```python
from build123d import *

# Parameters (mm, degrees)
F0_R     = 12.7
F1_DEPTH = 20.32
F2_T     = -2.54
F3_R     = 0.889


with BuildPart() as f1:
    # F0 (on Front) → F1 (new body)
    with BuildSketch(Plane.XZ):
        with Locations((37.7853997052, 47.8872768581)):
            Circle(F0_R)
    extrude(amount=F1_DEPTH)

    # F2
    f2_openings = [f1.faces().sort_by_distance(p)[0] for p in [
        (37.7854, -20.32, 47.887277),
    ]]
    offset(amount=F2_T, openings=f2_openings)

    # F3
    f3_edges = [f1.edges().sort_by_distance(p)[0] for p in [
        (25.0854, -20.32, 47.887277),
        (27.6254, -20.32, 47.887277),
    ]]
    fillet(f3_edges, radius=F3_R)


solid = f1.part
```
Part model, mm, in its own coordinate system. Give positions to 0.01 mm unless a question says otherwise; leave off trailing zeros. Loops run counter-clockwise (first coordinate to the right, second up) from the corner with the lowest first, then second, coordinate; pieces in that order, holes last. Notation, with made-up numbers: M 24,43 L 80,43 A11 ccw 80,59 Z; hole C -19.75,-26.5 d1. An arc over 180 degrees is marked long. Return JSON: item names as keys, results as strings.
1) Drill centre lines: line 1 (X direction, y = -13.25, z = 48); line 2 (Z direction, x = 38, y = -18.5); line 3 (Y direction, x = 41.25, z = 48). Where is each one in solid material? Low to high.
Calculated:
{"line 1": "x = 25.09 to 27.63, 47.94 to 50.48", "line 2": "z = 35.19 to 37.73, 58.05 to 60.59", "line 3": "y = -2.54 to 0"}
2) Flat gauge pins, fed straight in: pin 1 Ø1 at (x, z) = (44.5, 52) entering from -Y; pin 2 Ø2 at (y, z) = (-14.5, 55) entering from +X; pin 3 Ø1.5 at (x, z) = (33, 45.5) entering from +Y; pin 4 Ø2 at (x, y) = (47.5, -10) entering from +Z. Where does each tip first touch, or does it go through?
Calculated:
{"pin 1": "stops at y = -2.54", "pin 2": "stops at x = 48.92", "pin 3": "stops at y = 0", "pin 4": "stops at z = 57.13"}
3) Saw through at A-A, the plane y = -17.25. List the corners of the cut face in (x, z), then the cut area to 3 significant figures.
Calculated:
{"outline": "C 37.79,47.89 d25.4; hole C 37.79,47.89 d20.32", "area": "182 mm2"}
4) Pull direction X, two halves, no side cores. Call faces 1 (the face through (44.61, -9.58, 58.6)), 2 (the face through (42.47, -10.87, 38.87)), 3 (the face through (46, -20.32, 40)), 4 (the face through (38, -2.54, 48)): released by +X, released by -X, zero draft, split by the parting line, or undercut.
Calculated:
{"face 1": "split by the parting line", "face 2": "undercut", "face 3": "zero draft", "face 4": "undercut"}
